from build123d import *

# Parameters (mm, degrees)
F0_W     = 165
F0_H     = 5.432152
F0_H_2   = 85
F1_DEPTH = 5.08
F2_DEPTH = 13
F3_W     = 165
F3_H     = 5.479902
F4_DEPTH = 31.75
F6_DEPTH = 1.27


with BuildPart() as f1:
    # F0 (on Front) → F1 (new body)
    with BuildSketch(Plane.XZ):
        with Locations((0, 45.216076)):
            Rectangle(F0_W, F0_H)
        Rectangle(F0_W, F0_H_2)
        Polygon((82.5, 47.932152), (82.5, 42.5), (82.5, -42.5), (-82.5, -42.5), (-82.5, 42.5), (-82.5, 47.932152), (-88.101894, 47.932152), (-88.101894, -47.932152), (88.101894, -47.932152), (88.101894, 47.932152), align=None)
    extrude(amount=F1_DEPTH)

    # F0 (on Front) → F2 (join)
    with BuildSketch(Plane.XZ):
        Polygon((82.5, 47.932152), (82.5, 42.5), (82.5, -42.5), (-82.5, -42.5), (-82.5, 42.5), (-82.5, 47.932152), (-88.101894, 47.932152), (-88.101894, -47.932152), (88.101894, -47.932152), (88.101894, 47.932152), align=None)
    extrude(amount=-F2_DEPTH)

    # F3 (on face) → F4 (join)
    with BuildSketch(Plane(origin=(0, 13, 0), x_dir=(-1, 0, 0), z_dir=(0, 1, 0))):
        Polygon((82.5, 47.932152), (82.5, 42.45225), (82.5, -42.45225), (82.5, -42.5), (-82.5, -42.5), (-82.5, -42.45225), (-82.5, 42.45225), (-82.5, 47.932152), (-88.101894, 47.932152), (-88.101894, -47.932152), (88.101894, -47.932152), (88.101894, 47.932152), align=None)
        with Locations((0, 45.192201)):
            Rectangle(F3_W, F3_H)
    extrude(amount=F4_DEPTH)

    # F5 (on face) → F6 (join)
    with BuildSketch(Plane(origin=(82.5, 0, 0), x_dir=(0, -1, 0), z_dir=(-1, 0, 0))):
        Polygon((-13, -30.489394), (-13, 42.45225), (-14.72871, 42.45225), (-14.72871, -42.5), (-13, -42.5), align=None)
    extrude(amount=F6_DEPTH)


solid = f1.part
Verification items for the finished model (mm, model axes). A direction names the side the tool comes from. Give positions to 0.01 mm unless a question says otherwise; leave off trailing zeros. Loops run counter-clockwise (first coordinate to the right, second up) from the corner with the lowest first, then second, coordinate; pieces in that order, holes last.
1. Tool access check on faces 4 (the flat face through (0, 44.75, 43)), 5 (the flat face through (0, 13, 43)), 6 (the flat face through (-1, 22, -42.5)). Record the directions out of +Z, -Z, +X, -X, +Y, -Y that give a thin tool (end or side, any length) a straight path to the whole face; none if there is none.
Derived:
face 4: +Z, -Z, +X, -X, +Y
face 5: +Z
face 6: +Y
2. Cross-section at A-A on x = -6.5. Record the cut outline in (y, z).
Derived:
outline: (-5.08, -47.93) - (44.75, -47.93) - (44.75, -42.5) - (0, -42.5) - (0, 47.93) - (-5.08, 47.93) - close; (13, 42.45) - (44.75, 42.45) - (44.75, 47.93) - (13, 47.93) - close
3. Cross-section at C-C on z = -14.5. Record the cut outline in (x, y).
Derived:
outline: (-88.1, -5.08) - (88.1, -5.08) - (88.1, 44.75) - (82.5, 44.75) - (82.5, 14.73) - (81.23, 14.73) - (81.23, 13) - (82.5, 13) - (82.5, 0) - (-82.5, 0) - (-82.5, 44.75) - (-88.1, 44.75) - close
4. Release check for a two-part mould opening along Y. For faces 1 (the flat face through (82.5, 6, 2)), 2 (the flat face through (-1, -5.08, 1)), 3 (the flat face through (82.5, 30, -1)) record: +Y half, -Y half, draft (parallel to the pull), parting line (faces both ways), or undercut.
Derived:
face 1: undercut
face 2: -Y half
face 3: draft
5. Cross-section at B-B on y = 18. Record the cut outline in (x, z), and give its area (3 significant figures).
Derived:
outline: (-88.1, -47.93) - (88.1, -47.93) - (88.1, 47.93) - (-88.1, 47.93) - close; hole (-82.5, -42.5) - (82.5, -42.5) - (82.5, 42.45) - (-82.5, 42.45) - close
area: 2,870 mm2
6. Material ranges on probe 1 along X at (y, z) = (42, -12.5); probe 2 along Z at (x, y) = (70, 40); probe 3 along X at (y, z) = (14.5, 36), recorded low to high.
Derived:
probe 1: x = -88.1 to -82.5, 82.5 to 88.1
probe 2: z = -47.93 to -42.5, 42.45 to 47.93
probe 3: x = -88.1 to -82.5, 81.23 to 88.1
